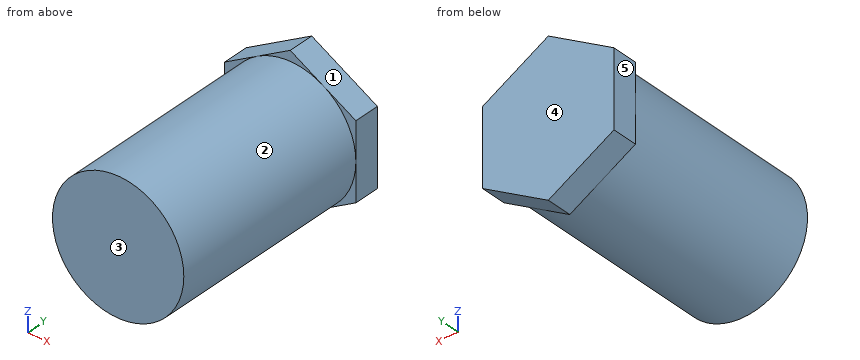
```python
from build123d import *

# Parameters (mm, degrees)
SKETCH1_R           = 12.5
BOSS_EXTRUDE1_DEPTH = 40
BOSS_EXTRUDE2_DEPTH = 5


with BuildPart() as part:
    # Sketch1 → Boss-Extrude1 (new body)
    with BuildSketch(Plane(origin=(0, 0, 0), x_dir=(1, 0, 0), z_dir=(0, 1, 0))):
        Circle(SKETCH1_R)
    extrude(amount=BOSS_EXTRUDE1_DEPTH)

    # Sketch2 → Boss-Extrude2 (add)
    with BuildSketch(Plane(origin=(0, 40, 0), x_dir=(1, 0, 0), z_dir=(0, 1, 0))):
        Polygon((0, -14.43375673), (12.5, -7.216878365), (12.5, 7.216878365), (0, 14.43375673), (-12.5, 7.216878365), (-12.5, -7.216878365), align=None)
    extrude(amount=BOSS_EXTRUDE2_DEPTH)


solid = part.part
```
Part model, mm, in its own coordinate system. Face numbers are marked on the shaded views. A direction names the side the tool comes from. Round coordinates to 2 decimals unless told otherwise and drop trailing zeros. Loops run counter-clockwise (first coordinate to the right, second up) from the corner with the lowest first, then second, coordinate; pieces in that order, holes last.
1. Slice it at A-A (y = 42). Give the cut face in (x, z), and give its area (3 significant figures).
Solutions:
outline: (-12.5, -7.22) - (0, -14.43) - (12.5, -7.22) - (12.5, 7.22) - (0, 14.43) - (-12.5, 7.22) - close
area: 541 mm2
2. 3-axis set-ups, long thin cutter, end or side, ignore diameter. For the marked faces 1 and 2: which of +Z, -Z, +X, -X, +Y, -Y reach the whole face in a straight line?
Solutions:
face 1: +Z, +X, +Y, -Y
face 2: -Y
3. Two-plate mould, pull along Y, no slides. Class the marked faces 3, 4 and 5: pulls with the +Y half, pulls with the -Y half, needs draft (parallel to the pull), parting line crosses it, or undercut.
Solutions:
face 3: pulls with the -Y half
face 4: pulls with the +Y half
face 5: needs draft
4. Flat gauge pins, fed straight in: pin 1 (10 mm diameter, centred on x = 5, y = 17.5, fed in from -Z); pin 2 (12 mm diameter, centred on y = 6, z = -8.5, fed in from -X); pin 3 (3 mm diameter, centred on x = 9, y = 38.5, fed in from +Z). Where does each tip first touch, or does it go through?
Solutions:
pin 1: stops at z = -12.5
pin 2: stops at x = -12.25
pin 3: stops at z = 10
5. Drill centre lines: line 1 along Z through (x, y) = (0.5, 10); line 2 along X through (y, z) = (28.5, 0.25); line 3 along X through (y, z) = (28.5, 7.25). Where is each one in solid material? Low to high.
Solutions:
line 1: z = -12.49 to 12.49
line 2: x = -12.5 to 12.5
line 3: x = -10.18 to 10.18
6. Slice it at D-D (y = 14.5). Give the cut face in (x, z), and give its area (3 significant figures).
Solutions:
outline: circle Ø25 at (0, 0)
area: 491 mm2
7. Slice it at B-B (x = 10.5). Give the cut face in (y, z), and give its area (3 significant figures).
Solutions:
outline: (0, -6.78) - (40, -6.78) - (40, -8.37) - (45, -8.37) - (45, 8.37) - (40, 8.37) - (40, 6.78) - (0, 6.78) - close
area: 626 mm2
8. Slice it at C-C (z = 9.75). Give the cut face in (x, y).
Solutions:
outline: (-8.11, 40) - (-7.82, 40) - (-7.82, 0) - (7.82, 0) - (7.82, 40) - (8.11, 40) - (8.11, 45) - (-8.11, 45) - close
